from build123d import *

# Parameters (mm, degrees)
F1_DEPTH = 320
F2_W     = 150
F2_H     = 26.066691
F3_DEPTH = 6


with BuildPart() as f1:
    # F0 (on Front) → F1 (new body)
    with BuildSketch(Plane.XZ):
        Polygon((-210, 0), (-210, -36.39128), (-204, -36.39128), (-204, -5.086953), (0, -5.086953), (204, -5.086953), (204, -36.39128), (210, -36.39128), (210, 0), (0, 0), align=None)
    extrude(amount=F1_DEPTH)

    # F2 (on face) → F3 (join)
    with BuildSketch(Plane.YZ.offset(210)):
        with Locations((-156.593922, 13.033345)):
            Rectangle(F2_W, F2_H)
    extrude(amount=-F3_DEPTH)


solid = f1.part
Model file for the job. Use its own axes, mm. A direction names the side the tool comes from. Coordinates: 2 decimals unless noted, no trailing zeros. Loops run counter-clockwise (first coordinate to the right, second up) from the corner with the lowest first, then second, coordinate; pieces in that order, holes last. Notation, with made-up numbers: (53.5, 10) -> (81.5, 10) arc R23 cw to (81.5, 24) -> close; hole circle Ø4 at (40.5, 59). An arc over 180 degrees is marked (long way). Use one line per item in the form item = value. Start each with the question number.
(1) Cut at A-A on y = -202.5. Give the cut face in (x, z).
(2) Cut at C-C on x = -16. Give the cut face in (y, z).
(3) Cut at D-D on z = 9. Give the cut face in (x, y), and give its area (3 significant figures).
(4) Probe probe 1 along X at (y, z) = (-243, -32.5); probe 2 along Z at (x, y) = (-75.5, -190); probe 3 along X at (y, z) = (-91, 4). List the from-to ranges inside material, lowest first. Write a range as from..to.
(5) Tool access for faces 5 (the flat face through (204, -158, -21)), 6 (the flat face through (-1, 0, -2)), 7 (the flat face through (204, -158, 13)): list every direction of +Z, -Z, +X, -X, +Y, -Y with a clear straight run to the whole face (end or side of a thin tool).
(6) Pull direction X, two halves, no side cores. Call faces 1 (the flat face through (-210, -158, -18)), 2 (the flat face through (-204, -158, -21)), 3 (the flat face through (-1, -320, -2)), 4 (the flat face through (-3, -158, -5.087)): pulls with the +X half, pulls with the -X half, needs draft (parallel to the pull), parting line crosses it, or undercut.
(7) Flat gauge pins, fed straight in: pin 1 (4 mm diameter, centred on y = -186, z = 4.5, fed in from -X); pin 2 (10 mm diameter, centred on x = -30, y = -69, fed in from +Z); pin 3 (10 mm diameter, centred on x = -28, z = -9.5, fed in from +Y); pin 4 (2 mm diameter, centred on x = -46, y = -285.5, fed in from -Z). Where does each tip first touch, or does it go through?
(8) Cut at B-B on z = -15.5. Give the cut face in (x, y).
Values:
q1.outline = (-210, -36.39) -> (-204, -36.39) -> (-204, -5.09) -> (204, -5.09) -> (204, -36.39) -> (210, -36.39) -> (210, 26.07) -> (204, 26.07) -> (204, 0) -> (-210, 0) -> close
q2.outline = (-320, -5.09) -> (0, -5.09) -> (0, 0) -> (-320, 0) -> close
q3.outline = (204, -231.59) -> (210, -231.59) -> (210, -81.59) -> (204, -81.59) -> close
q3.area = 900 mm2
q4.probe_1 = -210..-204, 204..210
q4.probe_2 = -5.09..0
q4.probe_3 = 204..210
q5.face_5 = -Z, +Y, -Y
q5.face_6 = +Z, -Z, +X, -X, +Y
q5.face_7 = +Z, -X, +Y, -Y
q6.face_1 = pulls with the -X half
q6.face_2 = undercut
q6.face_3 = needs draft
q6.face_4 = undercut
q7.pin_1 = 204
q7.pin_2 = 0
q7.pin_3 = 0
q7.pin_4 = -5.09
q8.outline = (-210, -320) -> (-204, -320) -> (-204, 0) -> (-210, 0) -> close; (204, -320) -> (210, -320) -> (210, 0) -> (204, 0) -> close
